CAD build for the part. Positions are in the model's coordinates, mm. A direction names the side the tool comes from. Coordinates: 2 decimals unless noted, no trailing zeros. Write each loop counter-clockwise with the first axis right and the second up, starting at its lowest first coordinate (ties: lowest second). Pieces come first, ordered by that corner, then holes.
```python
from build123d import *

# Parameters (mm, degrees)
CROQUIS1_W                 = 2.5
CROQUIS1_H                 = 13.5
SALIENTE_EXTRUIR1_DEPTH    = 4.5
CORTAR_EXTRUIR4_DEPTH      = 10
CORTAR_EXTRUIR4_DEPTH_BACK = 26.104780421
CROQUIS7_R                 = 0.875


with BuildPart() as part:
    # Croquis1 → Saliente-Extruir1 (new body)
    with BuildSketch(Plane(origin=(0, 0, 0), x_dir=(1, 0, 0), z_dir=(0, 1, 0))):
        with BuildLine():
            Line((-2, -10), (2, -10))
            ThreePointArc((2, -10), (4.121320344, -9.121320344), (5, -7))
            Line((5, -7), (5, 7))
            ThreePointArc((5, 7), (4.121320344, 9.121320344), (2, 10))
            Line((2, 10), (-2, 10))
            ThreePointArc((-2, 10), (-4.121320344, 9.121320344), (-5, 7))
            Line((-5, 7), (-5, 3))
            Line((-5, 3), (-21, 3))
            Line((-21, 3), (-21, 1))
            Line((-21, 1), (-5, 1))
            Line((-5, 1), (-5, -1))
            Line((-5, -1), (-21, -1))
            Line((-21, -1), (-21, -3))
            Line((-21, -3), (-5, -3))
            Line((-5, -3), (-5, -7))
            ThreePointArc((-5, -7), (-4.121320344, -9.121320344), (-2, -10))
        make_face()
        Rectangle(CROQUIS1_W, CROQUIS1_H, mode=Mode.SUBTRACT)
    extrude(amount=SALIENTE_EXTRUIR1_DEPTH)

    # Croquis7 → Cortar-Extruir4 (cut, two sides: drawn at the far end of the back side and taken through both)
    with BuildSketch(Plane.XY.offset(3).offset(-CORTAR_EXTRUIR4_DEPTH_BACK)):
        with Locations(Location((-19, 2.25, 0), (0, 0, 180))):
            Circle(CROQUIS7_R)
        with Locations(Location((-14.5, 2.25, 0), (0, 0, 180))):
            Circle(CROQUIS7_R)
    extrude(amount=CORTAR_EXTRUIR4_DEPTH + CORTAR_EXTRUIR4_DEPTH_BACK, mode=Mode.SUBTRACT)


solid = part.part
```
Item 1: Two-plate mould, pull along Z, no slides. Class faces 1 (the flat face through (-13, 2, 1)), 2 (the flat face through (-2, 0, 0)), 3 (the flat face through (0, 2, 10)): +Z half, -Z half, draft (parallel to the pull), parting line (faces both ways), or undercut.
Item 2: Saw through at B-B, the plane z = -4.5. Write the cut outline in (x, y), and give its area (4 significant figures).
Item 3: Flat gauge pins, fed straight in: pin 1 Ø1.5 at (x, y) = (-8.5, 4) entering from +Z; pin 2 Ø2 at (x, y) = (-15, 2.5) entering from -Z; pin 3 Ø1.6 at (x, y) = (-14.5, 2.25) entering from +Z; pin 4 Ø8 at (x, z) = (-8, 7.5) entering from +Y. Where does each tip first touch, or does it go through?
Item 4: Wall check: line 1 along X through (y, z) = (4.1, 4.5); line 2 along Z through (x, y) = (-19.5, 3.2); line 3 along Y through (x, z) = (-19, -1.6) (3 decimals). Give the ranges that are in metal, low to high.
Item 5: Saw through at A-A, the plane x = -6. Write the cut outline in (y, z), and give its area (3 significant figures).
Item 6: Which spindle directions (+Z, -Z, +X, -X, +Y, -Y) get a long thin tool onto all of the face, cutting with end or side? Do faces 4 (the flat face through (-5, 2, 5)), 5 (the flat face through (-13, 2, -3)), 6 (the flat face through (0, 2, -6.75)), 7 (the cylindrical face through (-19.8, 2.6, -2)), 8 (the flat face through (-13, 2, -1)). Say none if no direction does.
Item 7: Saw through at C-C, the plane y = 2.25. State how many separate pieces and enclosed holes the cut face has, and give its area (3 significant figures).
Item 8: Saw through at D-D, the plane x = -14.5. Write the cut outline in (y, z) (3 decimals).
Working result:
1. face 1: undercut
1. face 2: draft
1. face 3: +Z half
2. outline: (-5, 0) - (-1.25, 0) - (-1.25, 4.5) - (-5, 4.5) - close; (1.25, 0) - (5, 0) - (5, 4.5) - (1.25, 4.5) - close
2. area: 33.75 mm2
3. pin 1: stops at z = 3
3. pin 2: stops at z = -3
3. pin 3: passes through
3. pin 4: stops at y = 4.5
4. line 1: x = -5 to -1.25, 1.25 to 5
4. line 2: z = -3 to -1, 1 to 3
4. line 3: y = 0 to 1.375, 3.125 to 4.5
5. outline: (0, -3) - (4.5, -3) - (4.5, -1) - (0, -1) - close; (0, 1) - (4.5, 1) - (4.5, 3) - (0, 3) - close
5. area: 18.0 mm2
6. face 4: +Z, -X, +Y, -Y
6. face 5: -Z, -X, +Y, -Y
6. face 6: +Y, -Y
6. face 7: +Z, -Z
6. face 8: -X, +Y, -Y
7. separate pieces: 5
7. enclosed holes: 1
7. area: 209 mm2
8. outline: (0, -3) - (1.375, -3) - (1.375, -1) - (0, -1) - close; (0, 1) - (1.375, 1) - (1.375, 3) - (0, 3) - close; (3.125, -3) - (4.5, -3) - (4.5, -1) - (3.125, -1) - close; (3.125, 1) - (4.5, 1) - (4.5, 3) - (3.125, 3) - close
